The listing builds one solid part. Answer for the finished solid, in the listing's coordinates (mm). A direction names the side the tool comes from. Coordinates: 2 decimals unless noted, no trailing zeros. Loops run counter-clockwise (first coordinate to the right, second up) from the corner with the lowest first, then second, coordinate; pieces in that order, holes last. Notation, with made-up numbers: (88.5, -8.5) - (145.5, -8.5) arc R22 ccw to (145.5, -1.5) - close; hole circle Ø6 at (87.5, 14). An arc over 180 degrees is marked (long way). Put each result on its own line as item: value.
```python
from build123d import *

# Parameters (mm, degrees)
CUT_EXTRUDE_1_DEPTH = 25
CUT_EXTRUDE_2_DEPTH = 25


with BuildPart() as part:
    # Эскиз1 → Повернуть1 (revolve)
    with BuildSketch(Plane.XY):
        Polygon((0, 0), (17.5, 0), (17.5, -90), (26, -90), (14.05402905, -175), (0, -175), align=None)
    revolve(axis=Axis((0, 0, 0), (0, -1, 0)))

    # Эскиз2 → Вырез-Вытянуть1 (cut, symmetric)
    with BuildSketch(Plane.XY):
        with BuildLine():
            Line((10, -123), (10, -143))
            ThreePointArc((10, -143), (0, -153), (-10, -143))
            Line((-10, -143), (-10, -123))
            ThreePointArc((-10, -123), (0, -113), (10, -123))
        make_face()
    extrude(amount=CUT_EXTRUDE_1_DEPTH, both=True, mode=Mode.SUBTRACT)

    # Эскиз3 → Вырез-Вытянуть2 (cut)
    with BuildSketch(Plane(origin=(0, 0, 0), x_dir=(1, 0, 0), z_dir=(0, 1, 0))):
        with BuildLine():
            Line((-11, -13.610657589), (-11, 13.610657589))
            ThreePointArc((-11, 13.610657589), (-17.5, 0), (-11, -13.610657589))
        make_face()
        with BuildLine():
            ThreePointArc((17.5, 0), (15.791611697, 7.541551564), (11, 13.610657589))
            Line((11, 13.610657589), (11, -13.610657589))
            ThreePointArc((11, -13.610657589), (15.791611697, -7.541551564), (17.5, 0))
        make_face()
    extrude(amount=-CUT_EXTRUDE_2_DEPTH, mode=Mode.SUBTRACT)


solid = part.part
```
1) Straight lines are drawn through the part: L1, parallel to Y at x = -0.5, z = 11; L2, parallel to X at y = -13, z = -6; L3, parallel to Y at x = -13, z = 3. For each, find the intervals that lie inside material, in ascending order. Write a range as [from, to].
Found:
L1: y = [-175, -152.99], [-113.01, 0]
L2: x = [-11, 11]
L3: y = [-175, -25]
2) The part is cut by section A-A (x = 0). Give the vertices of the cut face in (y, z), and give its area (3 significant figures).
Found:
outline: (-175, -14.05) - (-153, -17.15) - (-153, 17.15) - (-175, 14.05) - close; (-113, -22.77) - (-90, -26) - (-90, -17.5) - (0, -17.5) - (0, 17.5) - (-90, 17.5) - (-90, 26) - (-113, 22.77) - close
area: 4,960 mm^2
3) Each of these flat-tipped pins is pushed along its axis until it touches: pin 1 (12 mm diameter, centred on x = -15.5, y = -50, fed in from +Z); pin 2 (1 mm diameter, centred on x = -8, y = -40.5, fed in from -Z); pin 3 (1 mm diameter, centred on x = 20.5, y = -102, fed in from -Z). Where does it stop, or does it pass through?
Found:
pin 1: stops at z = 14.7
pin 2: stops at z = -15.81
pin 3: stops at z = -13.84
4) The part is cut by section B-B (y = -136). Give the vertices of the cut face in (x, z).
Found:
outline: (-10, -16.78) - (-10, 16.78) arc R19.54 ccw to start; (10, -16.78) arc R19.54 ccw to (10, 16.78) - close
5) For faces 1 (the face through (16.69, -45.63, 5.26)), 2 (the face through (-10, -133, 0)), 3 (the face through (13, -25, 0)), determine the directions among +Z, -Z, +X, -X, +Y, -Y from which every point of the face is accessible in a straight line to the end or side of a thin tool.
Found:
face 1: +Y
face 2: +Z, -Z
face 3: +Z, -Z, +X, +Y
6) For a pull along X with two mould halves and no side action, classify faces 4 (the face through (-11, -12, 0)), 5 (the face through (0, -153, 0)), 6 (the face through (-14, -25, 0)) as pulls with the +X half, pulls with the -X half, needs draft (parallel to the pull), parting line crosses it, or undercut.
Found:
face 4: pulls with the -X half
face 5: undercut
face 6: needs draft
